Work out the finished part from the listing and answer in its coordinate system (mm). Round coordinates to 2 decimals unless told otherwise and drop trailing zeros. Write each loop counter-clockwise with the first axis right and the second up, starting at its lowest first coordinate (ties: lowest second). Pieces come first, ordered by that corner, then holes.
1. Find section C-C (y = 31.5). Write down the section's boundary in (x, z), and give its area (3 significant figures).
2. Straight lines are drawn through the part: probe 1 along Y at (x, z) = (-20, 0.25); probe 2 along Y at (x, z) = (8.5, 0.2); probe 3 along X at (y, z) = (29, 0.35). For each, find the intervals that lie inside material, in ascending order.
3. Find section D-D (y = -19.5). Write down the section's boundary in (x, z), and give its area (3 significant figures).
4. Find section B-B (z = 0.6). Write down the section's boundary in (x, y).
5. Find section A-A (x = -9). Write down the section's boundary in (y, z).
```python
from build123d import *

# Parameters (mm, degrees)
F0_W     = 150
F0_H     = 25
F1_DEPTH = 1


with BuildPart() as f1:
    # F0 (on Top) → F1 (new body)
    with BuildSketch(Plane.XY):
        with Locations((-75, 25.95)):
            Rectangle(F0_W, F0_H)
        with BuildLine():
            ThreePointArc((0, 13.45), (9.510586, 9.510586), (13.45, 0))
            ThreePointArc((13.45, 0), (9.510586, -9.510586), (0, -13.45))
            Line((0, -13.45), (0, -38.45))
            ThreePointArc((0, -38.45), (38.45, 0), (0, 38.45))
            Line((0, 38.45), (0, 13.45))
        make_face()
        with Locations((-75, -25.95)):
            Rectangle(F0_W, F0_H)
    extrude(amount=F1_DEPTH)


solid = f1.part
```
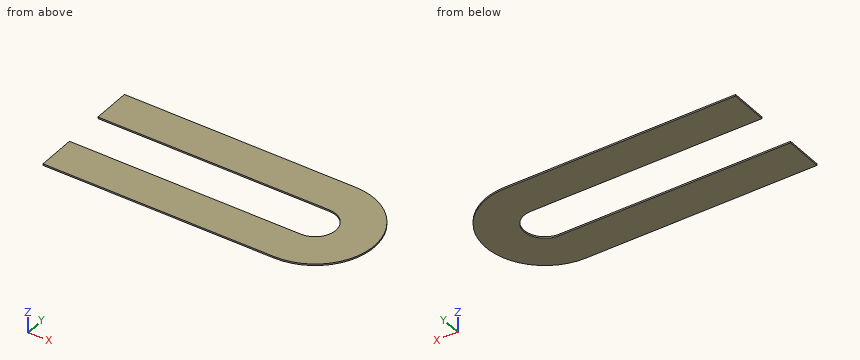
Worked answers:
1. outline: (-150, 0) - (22.05, 0) - (22.05, 1) - (-150, 1) - close
1. area: 172 mm2
2. probe 1: y = -38.45 to -13.45, 13.45 to 38.45
2. probe 2: y = -37.5 to -10.42, 10.42 to 37.5
2. probe 3: x = -150 to 25.25
3. outline: (-150, 0) - (33.14, 0) - (33.14, 1) - (-150, 1) - close
3. area: 183 mm2
4. outline: (-150, -38.45) - (0, -38.45) arc R38.45 ccw to (0, 38.45) - (-150, 38.45) - (-150, 13.45) - (0, 13.45) arc R13.45 cw to (13.45, 0) arc R13.45 cw to (0, -13.45) - (-150, -13.45) - close
5. outline: (-38.45, 0) - (-13.45, 0) - (-13.45, 1) - (-38.45, 1) - close; (13.45, 0) - (38.45, 0) - (38.45, 1) - (13.45, 1) - close
